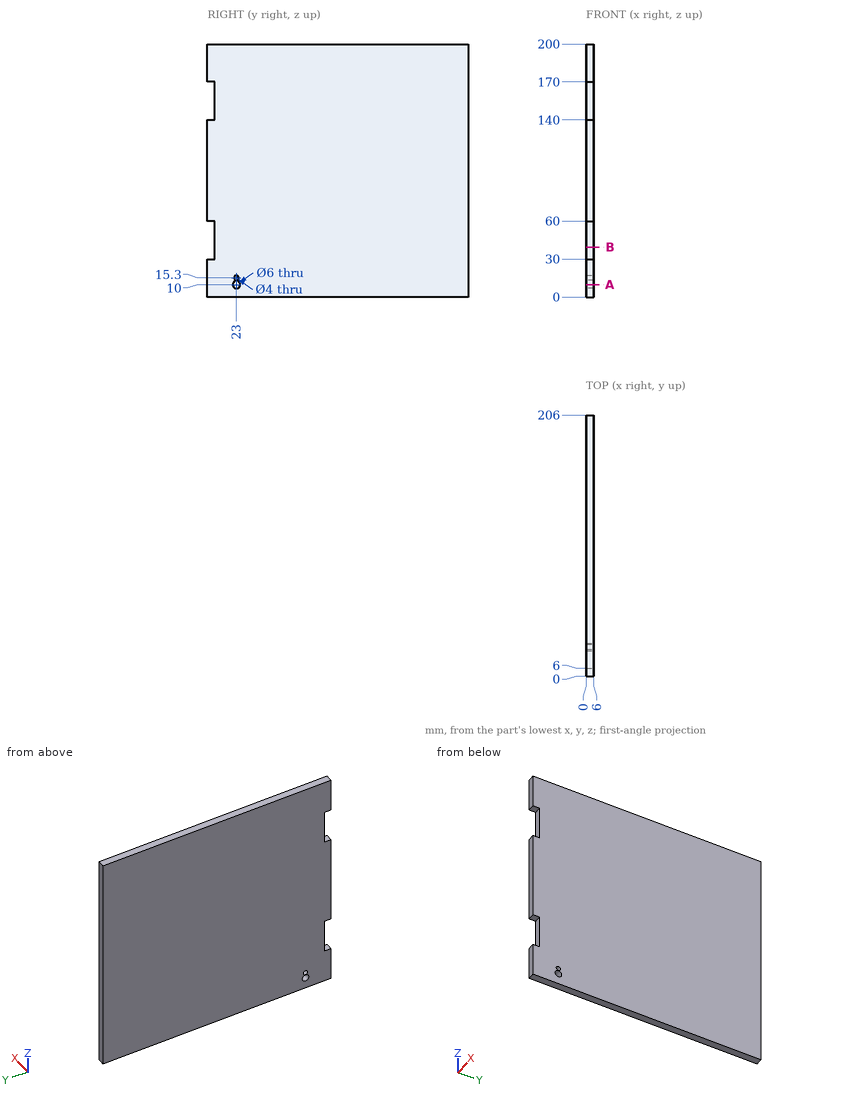
Could you check a few things on this drawing? It's one solid part, dimensions in mm from its lowest x, y, z. Coordinates: 2 decimals unless noted, no trailing zeros. Order: outer loops, then holes, each group sorted by start corner. A loop starts at its lowest first (then second) coordinate and runs counter-clockwise, first axis right, second up.
1) I need wall thicknesses on line 1 (Y direction, x = 2.6, z = 10); line 2 (Y direction, x = 1.4, z = 15.3); line 3 (Y direction, x = 2.1, z = 166.5). Which ranges of each line are inside material? Lowest first, please.
2) Imagine slicing it at A-A on z = 10. List the corners of the cut face in (x, y) for me.
3) Imagine slicing it at B-B on z = 39.5. List the corners of the cut face in (x, y) for me, and give its area (3 significant figures).
4) Will these pins go through, and if not, where does the flat tip stop? pin 1 (12 mm diameter, centred on y = 151.5, z = 69, fed in from -X); pin 2 (3 mm diameter, centred on x = 3, z = 152, fed in from -Y).
Response values:
1. line 1: y = 0 to 20, 26 to 206
1. line 2: y = 0 to 21, 25 to 206
1. line 3: y = 6 to 206
2. outline: (0, 0) - (6, 0) - (6, 20) - (0, 20) - close; (0, 26) - (6, 26) - (6, 206) - (0, 206) - close
3. outline: (0, 6) - (6, 6) - (6, 206) - (0, 206) - close
3. area: 1,200 mm2
4. pin 1: stops at x = 0
4. pin 2: stops at y = 6
